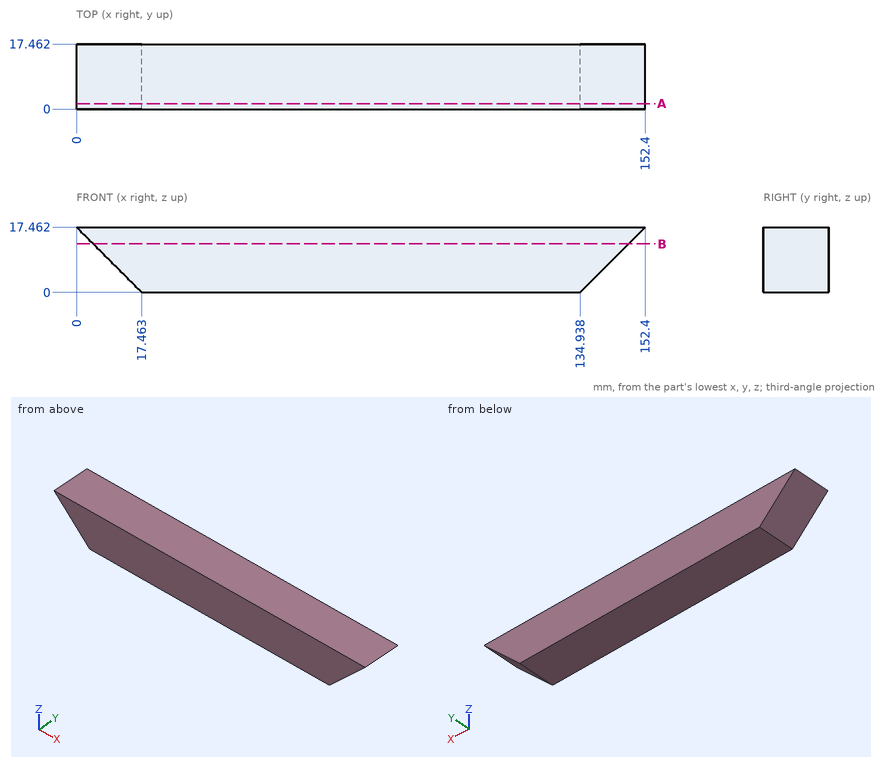
Study the drawing (mm; zero at the part's minimum x, y, z) and answer. Coordinates: 2 decimals unless noted, no trailing zeros. Loops run counter-clockwise (first coordinate to the right, second up) from the corner with the lowest first, then second, coordinate; pieces in that order, holes last. Notation, with made-up numbers: M 89,-8 L 141,-8 A12 ccw 141,13 Z; hole C -9.75,54 d1. An arc over 180 degrees is marked long. Answer in a Markdown table with one row per item. Add a question column.
1. Find section A-A, the plane y = 1.5. Write down the section's boundary in (x, z).
2. Flat-ended cylindrical pins translate along their axes: P1, Ø1, axis at x = 46, y = 3, coming from the -Z side; P2, Ø6, axis at y = 3.5, z = 2.5, coming from the +X side; P3, Ø2, axis at y = 15.5, z = 14, coming from the -X side; P4, Ø8, axis at y = 3.5, z = 12, coming from the -X side. Find the tip coordinate at first contact, or state that the pin passes through.
3. Find section B-B, the plane z = 13. Write down the section's boundary in (x, y).
4. Consider L1, parallel to X at y = 9.5, z = 13 (1 decimal); L2, parallel to X at y = 7.5, z = 7.5 (1 decimal). Determine where each line is inside the solid, lowest interval first.
Reported:
| question | item | result |
|---|---|---|
| 1 | outline | M 0,17.46 L 17.46,0 L 134.94,0 L 152.4,17.46 Z |
| 2 | P1 | stops at z = 0 |
| 2 | P2 | stops at x = 140.44 |
| 2 | P3 | stops at x = 2.46 |
| 2 | P4 | stops at x = 1.46 |
| 3 | outline | M 4.46,0 L 147.94,0 L 147.94,17.46 L 4.46,17.46 Z |
| 4 | L1 | x = 4.5 to 147.9 |
| 4 | L2 | x = 10 to 142.4 |
